Answer from the drawing. Dimensions are ordinates in mm from the lowest x, y and z of the part. Round coordinates to 2 decimals unless told otherwise and drop trailing zeros. Write each loop counter-clockwise with the first axis right and the second up, starting at its lowest first coordinate (ties: lowest second). Pieces come first, ordered by that corner, then holes. Notation, with made-up numbers: (24, -37.75) -> (35, -37.75) arc R14 cw to (35, -23.75) -> close; hole circle Ø6 at (-3, 86). An arc over 180 degrees is marked (long way). Return JSON: item names as keys, results as strings. Group by question number.
(1) Straight lines are drawn through the part: line 1 (Y direction, x = 2.5, z = 15.25); line 2 (Y direction, x = 20.5, z = 14.5); line 3 (X direction, y = 674.5, z = 14.25). For each, find the intervals that lie inside material, in ascending order.
(2) A cutting plane is placed at A-A on y = 340.5. Give the vertices of the cut face in (x, z).
(3) Given pin 1 (6.5 mm diameter, centred on y = 468.07, z = 15, fed in from +X) (3 decimals), flat-ended and moving along its own axis, determine where the tip first touches the part or whether it passes through.
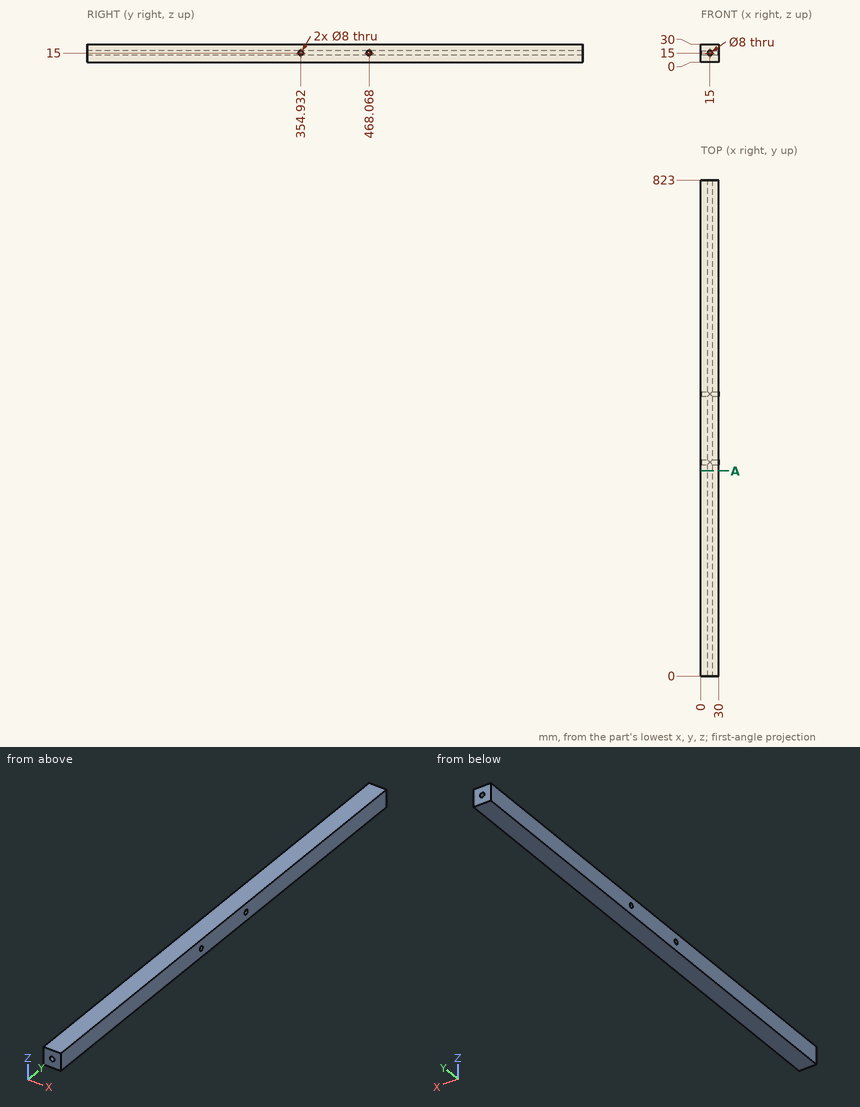
Checks:
{
 "1": {"line 1": "y = 0 to 350.94, 358.92 to 464.08, 472.06 to 823", "line 2": "y = 0 to 350.96, 358.9 to 464.1, 472.04 to 823", "line 3": "x = 0 to 11.07, 18.93 to 30"},
 "2": {"outline": "(0, 0) -> (30, 0) -> (30, 30) -> (0, 30) -> close; hole circle Ø8 at (15, 15)"},
 "3": {"pin 1": "passes through"}
}
